Model file for the job. Use its own axes, mm. A direction names the side the tool comes from. Round coordinates to 2 decimals unless told otherwise and drop trailing zeros. Write each loop counter-clockwise with the first axis right and the second up, starting at its lowest first coordinate (ties: lowest second). Pieces come first, ordered by that corner, then holes.
```python
from build123d import *

# Parameters (mm, degrees)
SKETCH1_W           = 77.75
SKETCH1_H           = 19.05
BOSS_EXTRUDE1_DEPTH = 2.54
SKETCH2_R           = 1.5875
CUT_EXTRUDE1_DEPTH  = 3.54
SKETCH3_W           = 49.022
SKETCH3_H           = 4.826
BOSS_EXTRUDE2_DEPTH = 4.4958
SKETCH4_W           = 45.974
SKETCH4_H           = 1.7018
CUT_EXTRUDE2_DEPTH  = 4.4958
SKETCH6_W           = 40.810788913
SKETCH6_H           = 1.5621
CUT_EXTRUDE3_DEPTH  = 4.4958


with BuildPart() as part:
    # Sketch1 → Boss-Extrude1 (new body)
    with BuildSketch(Plane(origin=(0, 0, 0), x_dir=(1, 0, 0), z_dir=(0, 1, 0))):
        Rectangle(SKETCH1_W, SKETCH1_H)
    extrude(amount=BOSS_EXTRUDE1_DEPTH)

    # Sketch2 → Cut-Extrude1 (cut, through all)
    with BuildSketch(Plane(origin=(0, 2.54, 0), x_dir=(1, 0, 0), z_dir=(0, 1, 0))):
        with Locations((35.2047, 0)):
            Circle(SKETCH2_R)
        with Locations((-35.2047, 0)):
            Circle(SKETCH2_R)
    extrude(amount=-CUT_EXTRUDE1_DEPTH, mode=Mode.SUBTRACT)

    # Sketch3 → Boss-Extrude2 (add)
    with BuildSketch(Plane(origin=(0, 2.54, 0), x_dir=(1, 0, 0), z_dir=(0, 1, 0))):
        Rectangle(SKETCH3_W, SKETCH3_H)
    extrude(amount=BOSS_EXTRUDE2_DEPTH)

    # Sketch4 → Cut-Extrude2 (cut)
    with BuildSketch(Plane(origin=(0, 7.0358, 0), x_dir=(1, 0, 0), z_dir=(0, 1, 0))):
        Rectangle(SKETCH4_W, SKETCH4_H)
    extrude(amount=-CUT_EXTRUDE2_DEPTH, mode=Mode.SUBTRACT)

    # Sketch6 → Cut-Extrude3 (cut)
    with BuildSketch(Plane(origin=(0, 7.0358, 0), x_dir=(1, 0, 0), z_dir=(0, 1, 0))):
        with Locations((-0.321005544, -1.63195)):
            Rectangle(SKETCH6_W, SKETCH6_H)
        with Locations((-0.321005544, 1.63195)):
            Rectangle(SKETCH6_W, SKETCH6_H)
    extrude(amount=-CUT_EXTRUDE3_DEPTH, mode=Mode.SUBTRACT)


solid = part.part
```
1) Cut at B-B on y = 6.25. List the corners of the cut face in (x, z), and give its area (3 significant figures).
2) Cut at D-D on x = 27.5. List the corners of the cut face in (y, z) (3 decimals).
3) Cut at A-A on z = 0. List the corners of the cut face in (x, y) (3 decimals), and give its area (3 significant figures).
4) Flat gauge pins, fed straight in: pin 1 Ø1.4 at (y, z) = (5, 0.5) entering from +X; pin 2 Ø0.7 at (x, y) = (-22, 5) entering from -Z; pin 3 Ø3.5 at (y, z) = (5.5, 0) entering from -X; pin 4 Ø3 at (x, z) = (-35.2, 0) entering from +Y. Where does each tip first touch, or does it go through?
5) Which spindle directions (+Z, -Z, +X, -X, +Y, -Y) get a long thin tool onto all of the face, cutting with end or side? Do faces 1 (the face through (-23, 5, 2.413)), 2 (the face through (20.084, 5, -2)), 3 (the face through (22.987, 5, 0)). Say none if no direction does.
6) Pull direction X, two halves, no side cores. Call faces 4 (the face through (22, 5, -0.851)), 5 (the face through (24.511, 5, 0)), 6 (the face through (-1, 0, 0)): released by +X, released by -X, zero draft, split by the parting line, or undercut.
7) Wall check: probe 1 along X at (y, z) = (1, 0) (3 decimals); probe 2 along X at (y, z) = (3.5, 2); probe 3 along Z at (x, y) = (-22, 5.5). Give the ranges that are in metal, low to high.
8) Cut at C-C on z = -4. List the corners of the cut face in (x, y) (3 decimals).
Result sheet:
1. outline: (-24.51, -2.41) - (-20.73, -2.41) - (-20.73, -0.85) - (-22.99, -0.85) - (-22.99, 0.85) - (-20.73, 0.85) - (-20.73, 2.41) - (-24.51, 2.41) - close; (20.08, -2.41) - (24.51, -2.41) - (24.51, 2.41) - (20.08, 2.41) - (20.08, 0.85) - (22.99, 0.85) - (22.99, -0.85) - (20.08, -0.85) - close
1. area: 30.8 mm2
2. outline: (0, -9.525) - (2.54, -9.525) - (2.54, 9.525) - (0, 9.525) - close
3. outline: (-38.875, 0) - (-36.792, 0) - (-36.792, 2.54) - (-38.875, 2.54) - close; (-33.617, 0) - (33.617, 0) - (33.617, 2.54) - (24.511, 2.54) - (24.511, 7.036) - (22.987, 7.036) - (22.987, 2.54) - (-22.987, 2.54) - (-22.987, 7.036) - (-24.511, 7.036) - (-24.511, 2.54) - (-33.617, 2.54) - close; (36.792, 0) - (38.875, 0) - (38.875, 2.54) - (36.792, 2.54) - close
3. area: 195 mm2
4. pin 1: stops at x = 24.51
4. pin 2: stops at z = -2.41
4. pin 3: stops at x = -24.51
4. pin 4: passes through
5. face 1: +Z, +X, -X, +Y
5. face 2: +Z, -Z, +Y
5. face 3: +Y
6. face 4: undercut
6. face 5: released by +X
6. face 6: zero draft
7. probe 1: x = -38.875 to -36.792, -33.617 to 33.617, 36.792 to 38.875
7. probe 2: x = -24.51 to -20.73, 20.08 to 24.51
7. probe 3: z = -2.41 to -0.85, 0.85 to 2.41
8. outline: (-38.875, 0) - (38.875, 0) - (38.875, 2.54) - (-38.875, 2.54) - close
